from build123d import *

# Parameters (mm, degrees)
S01_M6_THREADED_SHANK_R                  = 3
F_01_M6_THREADED_SHANK_DEPTH             = 16
F_02_START                               = -1.2
S02_BUTTON_HEAD_CLEARING_DIAMETER_R      = 5.25
F_02_BUTTON_HEAD_CLEARING_DIAMETER_DEPTH = 1.2
F_03_START                               = -3.3
S03_BUTTON_CROWN_R                       = 4.3
F_03_BUTTON_CROWN_DEPTH                  = 2.1
F_04_START                               = -3.4
F_04_4_MM_HEX_SOCKET_DEPTH               = 2.2


with BuildPart() as part:
    # S01 - M6 threaded shank → 01 - M6 threaded shank (new body)
    with BuildSketch(Plane.XY):
        Circle(S01_M6_THREADED_SHANK_R)
    extrude(amount=F_01_M6_THREADED_SHANK_DEPTH)

    # S02 - Button head clearing diameter → 02 - Button head clearing diameter (add)
    with BuildSketch(Plane.XY.offset(F_02_START)):
        Circle(S02_BUTTON_HEAD_CLEARING_DIAMETER_R)
    extrude(amount=F_02_BUTTON_HEAD_CLEARING_DIAMETER_DEPTH)

    # S03 - Button crown → 03 - Button crown (add)
    with BuildSketch(Plane.XY.offset(F_03_START)):
        Circle(S03_BUTTON_CROWN_R)
    extrude(amount=F_03_BUTTON_CROWN_DEPTH)

    # S04 - 4 mm hex socket → 04 - 4 mm hex socket (cut)
    with BuildSketch(Plane.XY.offset(F_04_START)):
        Polygon((2.309401077, 0), (1.154700538, 2), (-1.154700538, 2), (-2.309401077, 0), (-1.154700538, -2), (1.154700538, -2), align=None)
    extrude(amount=F_04_4_MM_HEX_SOCKET_DEPTH, mode=Mode.SUBTRACT)


solid = part.part
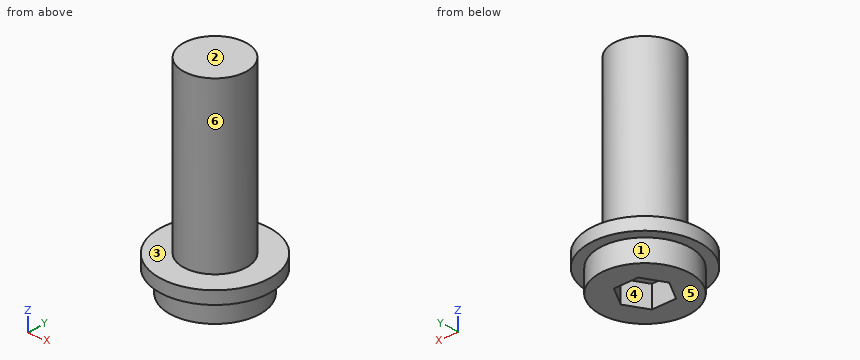
Geometry check sheet. Reference: the model listing, model coordinates, mm. Face numbers are marked on the shaded views. A direction names the side the tool comes from. Round coordinates to 2 decimals unless told otherwise and drop trailing zeros. Loops run counter-clockwise (first coordinate to the right, second up) from the corner with the lowest first, then second, coordinate; pieces in that order, holes last. Notation, with made-up numbers: (13.25, 85.5) - (35.25, 85.5) arc R19 ccw to (35.25, 94.5) - close; hole circle Ø10 at (81, -37). An arc over 180 degrees is marked (long way). One line per question, with ' | ' between items. Start each with the question number.
1. Tool access check on the marked faces 1, 2 and 3. Record the directions out of +Z, -Z, +X, -X, +Y, -Y that give a thin tool (end or side, any length) a straight path to the whole face; none if there is none.
2. Cross-section at A-A on x = 0. Record the cut outline in (y, z), then the cut area to 3 significant figures.
3. Scan lines: line 1 (Z direction, x = -3.5, y = -1); line 2 (Z direction, x = 4.25, y = -2.25); line 3 (Y direction, x = -2, z = 2.25). Record each from-to range of solid material in increasing order. Write a range as [from, to].
4. Cross-section at B-B on y = -1.75. Record the cut outline in (x, z), then the cut area to 3 significant figures.
5. Cross-section at C-C on z = -0.5. Record the cut outline in (x, y), then the cut area to 3 significant figures.
6. Draft check along X on the marked faces 4, 5 and 6. Enter one of: released by +X, released by -X, zero draft, split by the parting line, or undercut.
7. Cross-section at D-D on z = 7.75. Record the cut outline in (x, y), then the cut area to 3 significant figures.
8. Depth check by flat-ended pin: pin 1 (1 mm diameter, centred on x = 0, z = -2.5, fed in from -Y); pin 2 (6 mm diameter, centred on y = 0.5, z = 12.5, fed in from -X); pin 3 (0.6 mm diameter, centred on x = 0.5, z = -2.5, fed in from +Y). Enter the tip coordinate at first touch or a pass-through.
Taken from the geometry:
1) face 1: -Z | face 2: +Z, +X, -X, +Y, -Y | face 3: +Z
2) outline: (-5.25, -1.2) - (-4.3, -1.2) - (-4.3, -3.3) - (-2, -3.3) - (-2, -1.2) - (2, -1.2) - (2, -3.3) - (4.3, -3.3) - (4.3, -1.2) - (5.25, -1.2) - (5.25, 0) - (3, 0) - (3, 16) - (-3, 16) - (-3, 0) - (-5.25, 0) - close | area: 118 mm²
3) line 1: [-3.3, 0] | line 2: [-1.2, 0] | line 3: [-2.24, 2.24]
4) outline: (-4.95, -1.2) - (-3.93, -1.2) - (-3.93, -3.3) - (-1.3, -3.3) - (-1.3, -1.2) - (1.3, -1.2) - (1.3, -3.3) - (3.93, -3.3) - (3.93, -1.2) - (4.95, -1.2) - (4.95, 0) - (2.44, 0) - (2.44, 16) - (-2.44, 16) - (-2.44, 0) - (-4.95, 0) - close | area: 101 mm²
5) outline: circle Ø10.5 at (0, 0) | area: 86.6 mm²
6) face 4: undercut | face 5: zero draft | face 6: split by the parting line
7) outline: circle Ø6 at (0, 0) | area: 28.3 mm²
8) pin 1: y = -4.3 | pin 2: x = -3 | pin 3: y = 4.3
